CAD build for the part. Positions are in the model's coordinates, mm. Give positions to 0.01 mm unless a question says otherwise; leave off trailing zeros. Order: outer loops, then holes, each group sorted by start corner. A loop starts at its lowest first (then second) coordinate and runs counter-clockwise, first axis right, second up.
Item 1: Band-saw the part on B-B on x = 3. Give the cut face in (y, z), plus the area to 3 significant figures.
Item 2: Band-saw the part on A-A on y = 32.5. Give the cut face in (x, z) (3 decimals), plus the area to 3 significant figures.
Item 3: Flat gauge pins, fed straight in: P1, Ø2.5, axis at x = 3, y = 62, coming from the +Z side; P2, Ø5, axis at x = 3, y = 3, coming from the -Z side. Where does each tip first touch, or does it go through?
Item 4: Band-saw the part on D-D on x = 103.5. Give the cut face in (y, z).
Item 5: Wall check: L1, parallel to Y at x = 157, z = 0.5; L2, parallel to X at y = 27.5, z = 0.45; L3, parallel to Y at x = 110, z = 0.2. Give the ranges that are in metal, low to high.
Item 6: Band-saw the part on C-C on z = 0.7. Give the cut face in (x, y) (3 decimals).
```python
from build123d import *

# Parameters (mm, degrees)
ESQUISSE1_W             = 160
ESQUISSE1_H             = 65
ESQUISSE1_R             = 1.5
BOSS_EXTRU_1_DEPTH      = 0.9
ESQUISSE2_R             = 2
ESQUISSE2_W             = 85
ESQUISSE2_H             = 50
ENL_V_MAT_EXTRU_1_DEPTH = 0.9


with BuildPart() as part:
    # Esquisse1 → Boss.-Extru.1 (new body)
    with BuildSketch(Plane.XY):
        with Locations((80, 32.5)):
            Rectangle(ESQUISSE1_W, ESQUISSE1_H)
        with Locations((3, 62)):
            Circle(ESQUISSE1_R, mode=Mode.SUBTRACT)
        with Locations((3, 3)):
            Circle(ESQUISSE1_R, mode=Mode.SUBTRACT)
        with Locations((157, 3)):
            Circle(ESQUISSE1_R, mode=Mode.SUBTRACT)
        with Locations((157, 62)):
            Circle(ESQUISSE1_R, mode=Mode.SUBTRACT)
    extrude(amount=BOSS_EXTRU_1_DEPTH)

    # Esquisse2 → Enlèv. mat.-Extru.1 (cut)
    with BuildSketch(Plane.XY.offset(0.9)):
        with Locations((33.825, 32.5)):
            Circle(ESQUISSE2_R)
        with Locations((126.175, 32.5)):
            Circle(ESQUISSE2_R)
        with Locations((80, 32.5)):
            Rectangle(ESQUISSE2_W, ESQUISSE2_H)
    extrude(amount=-ENL_V_MAT_EXTRU_1_DEPTH, mode=Mode.SUBTRACT)


solid = part.part
```
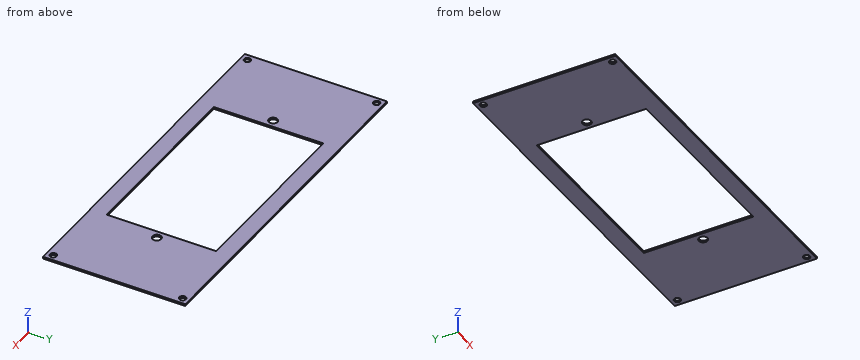
The answers:
1. outline: (0, 0) - (1.5, 0) - (1.5, 0.9) - (0, 0.9) - close; (4.5, 0) - (60.5, 0) - (60.5, 0.9) - (4.5, 0.9) - close; (63.5, 0) - (65, 0) - (65, 0.9) - (63.5, 0.9) - close
1. area: 53.1 mm2
2. outline: (0, 0) - (31.825, 0) - (31.825, 0.9) - (0, 0.9) - close; (35.825, 0) - (37.5, 0) - (37.5, 0.9) - (35.825, 0.9) - close; (122.5, 0) - (124.175, 0) - (124.175, 0.9) - (122.5, 0.9) - close; (128.175, 0) - (160, 0) - (160, 0.9) - (128.175, 0.9) - close
2. area: 60.3 mm2
3. P1: passes through
3. P2: stops at z = 0
4. outline: (0, 0) - (7.5, 0) - (7.5, 0.9) - (0, 0.9) - close; (57.5, 0) - (65, 0) - (65, 0.9) - (57.5, 0.9) - close
5. L1: y = 0 to 1.5, 4.5 to 60.5, 63.5 to 65
5. L2: x = 0 to 37.5, 122.5 to 160
5. L3: y = 0 to 7.5, 57.5 to 65
6. outline: (0, 0) - (160, 0) - (160, 65) - (0, 65) - close; hole circle Ø3 at (3, 3); hole circle Ø3 at (3, 62); hole circle Ø4 at (33.825, 32.5); hole (37.5, 7.5) - (122.5, 7.5) - (122.5, 57.5) - (37.5, 57.5) - close; hole circle Ø4 at (126.175, 32.5); hole circle Ø3 at (157, 3); hole circle Ø3 at (157, 62)
